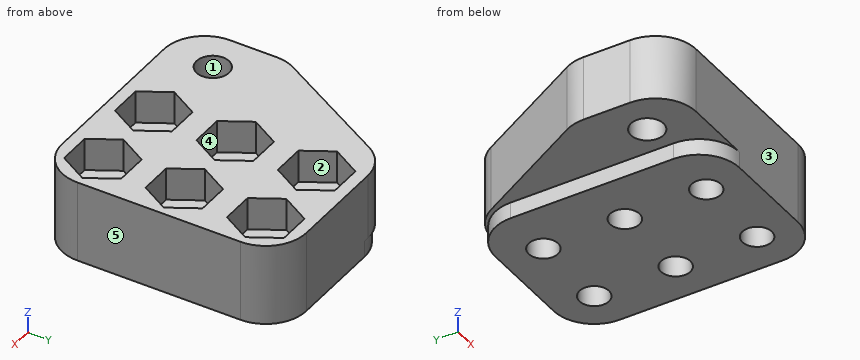
```python
from build123d import *

# Parameters (mm, degrees)
SKETCH1_R           = 2.286
SKETCH1_R_2         = 2.54
BOSS_EXTRUDE1_DEPTH = 12.7
FILLET1_R           = 6.35
CUT_EXTRUDE1_DEPTH  = 5.08
CUT_EXTRUDE2_START  = -2.54
SKETCH3_R           = 2.54
CUT_EXTRUDE2_DEPTH  = 2.54
FILLET2_R           = 6.35


with BuildPart() as part:
    # Sketch1 → Boss-Extrude1 (new body)
    with BuildSketch(Plane.XY):
        Polygon((-6.35, 31.75), (-19.05, 8.89), (-19.05, -6.35), (-6.35, -6.35), (19.05, -6.35), (19.05, 31.75), align=None)
        Circle(SKETCH1_R, mode=Mode.SUBTRACT)
        with Locations((-12.7, 1.27)):
            Circle(SKETCH1_R_2, mode=Mode.SUBTRACT)
        with Locations((12.7, 0)):
            Circle(SKETCH1_R, mode=Mode.SUBTRACT)
        with Locations((12.7, 12.7)):
            Circle(SKETCH1_R, mode=Mode.SUBTRACT)
        with Locations((12.7, 25.4)):
            Circle(SKETCH1_R, mode=Mode.SUBTRACT)
        with Locations((0, 12.7)):
            Circle(SKETCH1_R, mode=Mode.SUBTRACT)
        with Locations((0, 25.4)):
            Circle(SKETCH1_R, mode=Mode.SUBTRACT)
    extrude(amount=BOSS_EXTRUDE1_DEPTH)

    # Fillet1
    fillet1_edges = [part.edges().sort_by_distance(p)[0] for p in [
        (-19.05, -6.35, 6.35),
        (-19.05, 8.89, 6.35),
        (-6.35, 31.75, 6.35),
        (19.05, 31.75, 6.35),
        (19.05, -6.35, 6.35),
    ]]
    fillet(fillet1_edges, radius=FILLET1_R)

    # Sketch2 → Cut-Extrude1 (cut)
    with BuildSketch(Plane.XY.offset(12.7)):
        Polygon((17.832643893, 0), (15.266321947, 4.445), (10.133678053, 4.445), (7.567356107, 0), (10.133678053, -4.445), (15.266321947, -4.445), align=None)
        Polygon((5.132643893, 0), (2.566321947, 4.445), (-2.566321947, 4.445), (-5.132643893, 0), (-2.566321947, -4.445), (2.566321947, -4.445), align=None)
        Polygon((17.832643893, 12.7), (15.266321947, 17.145), (10.133678053, 17.145), (7.567356107, 12.7), (10.133678053, 8.255), (15.266321947, 8.255), align=None)
        Polygon((17.832643893, 25.4), (15.266321947, 29.845), (10.133678053, 29.845), (7.567356107, 25.4), (10.133678053, 20.955), (15.266321947, 20.955), align=None)
        Polygon((5.132643893, 12.7), (2.566321947, 17.145), (-2.566321947, 17.145), (-5.132643893, 12.7), (-2.566321947, 8.255), (2.566321947, 8.255), align=None)
        Polygon((5.132643893, 25.4), (2.566321947, 29.845), (-2.566321947, 29.845), (-5.132643893, 25.4), (-2.566321947, 20.955), (2.566321947, 20.955), align=None)
    extrude(amount=-CUT_EXTRUDE1_DEPTH, mode=Mode.SUBTRACT)

    # Sketch3 → Cut-Extrude2 (cut)
    with BuildSketch(Plane(origin=(0, 0, 0), x_dir=(-1, 0, 0), z_dir=(0, 0, -1)).offset(CUT_EXTRUDE2_START)):
        with BuildLine():
            Line((18.250898703, 10.328382334), (8.164537437, 28.483832613))
            Line((8.164537437, 28.483832613), (8.164537437, -6.35))
            Line((8.164537437, -6.35), (12.7, -6.35))
            ThreePointArc((12.7, -6.35), (17.190128061, -4.490128061), (19.05, 0))
            Line((19.05, 0), (19.05, 7.244549721))
            ThreePointArc((19.05, 7.244549721), (18.846979208, 8.837392029), (18.250898703, 10.328382334))
        make_face()
        with Locations((12.7, 1.27)):
            Circle(SKETCH3_R, mode=Mode.SUBTRACT)
    extrude(amount=CUT_EXTRUDE2_DEPTH, mode=Mode.SUBTRACT)

    # Fillet2
    # the kernel refuses this fillet: 6.35 mm, written as the material it takes off along each edge
    with BuildSketch(Plane(origin=(-8.164537437, -6.35, 2.54), x_dir=(1, 0, 0), z_dir=(0, 0, -1))) as fillet2_piece_1:
        with BuildLine():
            CenterArc((FILLET2_R, -FILLET2_R), FILLET2_R, 90, 90)
            Line((0, -FILLET2_R), (0, 0))
            Line((0, 0), (FILLET2_R, 0))
        make_face()
    extrude(amount=18.415, mode=Mode.SUBTRACT)
    with BuildSketch(Plane(origin=(-8.164537437, 28.483832613, -17.851881799), x_dir=(0.8892619937285123, 0.45739819250844366, 0), z_dir=(0, 0, 1))) as fillet2_piece_2:
        with BuildLine():
            CenterArc((4.236274197, -5.64681366), FILLET2_R, 62.780655364, 90)
            Line((-1.410539463, -2.742335138), (-1.975220829, -2.451887286))
            Line((-1.975220829, -2.451887286), (-0.564681366, 0.290447852))
            Line((-0.564681366, 0.290447852), (-0.352566378, 0.528130617))
            ThreePointArc((-0.352566378, 0.528130617), (6.720590159, 0.930188855), (7.431200572, 0.564681366))
            Line((7.431200572, 0.564681366), (7.140752719, 0))
        make_face()
    extrude(amount=20.391881799, mode=Mode.SUBTRACT)


solid = part.part
```
Verification items for the finished model (mm, model axes). Face numbers are marked on the shaded views. A direction names the side the tool comes from. Coordinates: 2 decimals unless noted, no trailing zeros. Order: outer loops, then holes, each group sorted by start corner. A loop starts at its lowest first (then second) coordinate and runs counter-clockwise, first axis right, second up. Notation, with made-up numbers: (14, 59.5) - (36, 59.5) arc R20 cw to (36, 86.5) - close; hole circle Ø2 at (64, 38.25). An arc over 180 degrees is marked (long way). Return JSON: item names as keys, results as strings.
(1) Go/stop test with flat-tipped pins: pin 1 (1 mm diameter, centred on y = 13.5, z = 7.5, fed in from -X); pin 2 (6 mm diameter, centred on x = 0, y = 12.7, fed in from +Z); pin 3 (0.8 mm diameter, centred on y = 9.5, z = 1.5, fed in from -X). Record where each tip stops, or that it passes through.
Filled sheet:
{"pin 1": "stops at x = -16.77", "pin 2": "stops at z = 7.62", "pin 3": "stops at x = -8.16"}
(2) Access from +Z, -Z, +X, -X, +Y, -Y to the whole of each face (thin tool, end or side, straight path). Record for the marked faces 1 and 2.
Filled sheet:
{"face 1": "+Z, -Z", "face 2": "+Z"}
(3) Section check B-B, the plane y = 13.5. Record the cut outline in (x, z), and give its area (3 significant figures).
Filled sheet:
{"outline": "(-16.49, 2.54) - (-8.16, 2.54) - (-8.16, 0) - (-2.14, 0) - (-2.14, 7.62) - (-4.67, 7.62) - (-4.67, 12.7) - (-16.49, 12.7) - close; (2.14, 0) - (10.56, 0) - (10.56, 7.62) - (8.03, 7.62) - (8.03, 12.7) - (4.67, 12.7) - (4.67, 7.62) - (2.14, 7.62) - close; (14.84, 0) - (19.05, 0) - (19.05, 12.7) - (17.37, 12.7) - (17.37, 7.62) - (14.84, 7.62) - close", "area": "270 mm^2"}
(4) Mould release check, pull along Y, two halves, no side actions. Record for the marked faces 3, 4 and 5: pulls with the +Y half, pulls with the -Y half, needs draft (parallel to the pull), parting line crosses it, or undercut.
Filled sheet:
{"face 3": "pulls with the -Y half", "face 4": "undercut", "face 5": "needs draft"}
(5) Thickness scan on line 1 along Y through (x, z) = (0, 2); line 2 along X through (y, z) = (12.7, 4); line 3 along X through (y, z) = (26.5, 0.75). Record the ranges inside material, lowest first.
Filled sheet:
{"line 1": "y = -6.35 to -2.29, 2.29 to 10.41, 14.99 to 23.11, 27.69 to 31.75", "line 2": "x = -16.93 to -2.29, 2.29 to 10.41, 14.99 to 19.05", "line 3": "x = -8.07 to -2, 2 to 10.7, 14.7 to 18.95"}
(6) Section check C-C, the plane z = 1.75. Record the cut outline in (x, y).
Filled sheet:
{"outline": "(-8.16, 0) arc R6.35 ccw to (-1.81, -6.35) - (12.7, -6.35) arc R6.35 ccw to (19.05, 0) - (19.05, 25.4) arc R6.35 ccw to (12.7, 31.75) - (-1.81, 31.75) arc R6.35 ccw to (-8.16, 25.4) - close; hole circle Ø4.57 at (0, 0); hole circle Ø4.57 at (0, 12.7); hole circle Ø4.57 at (0, 25.4); hole circle Ø4.57 at (12.7, 0); hole circle Ø4.57 at (12.7, 12.7); hole circle Ø4.57 at (12.7, 25.4)"}
(7) Section check A-A, the plane z = 5.75. Record the cut outline in (x, y).
Filled sheet:
{"outline": "(-19.05, 0) arc R6.35 ccw to (-12.7, -6.35) - (12.7, -6.35) arc R6.35 ccw to (19.05, 0) - (19.05, 25.4) arc R6.35 ccw to (12.7, 31.75) - (-2.61, 31.75) arc R6.35 ccw to (-8.16, 28.48) - (-18.25, 10.33) arc R6.35 ccw to (-19.05, 7.24) - close; hole circle Ø5.08 at (-12.7, 1.27); hole circle Ø4.57 at (0, 0); hole circle Ø4.57 at (0, 12.7); hole circle Ø4.57 at (0, 25.4); hole circle Ø4.57 at (12.7, 0); hole circle Ø4.57 at (12.7, 12.7); hole circle Ø4.57 at (12.7, 25.4)"}
(8) Section check D-D, the plane x = 11. Record the cut outline in (y, z) (3 decimals).
Filled sheet:
{"outline": "(-6.35, 0) - (-1.528, 0) - (-1.528, 7.62) - (-4.445, 7.62) - (-4.445, 12.7) - (-6.35, 12.7) - close; (1.528, 0) - (11.172, 0) - (11.172, 7.62) - (8.255, 7.62) - (8.255, 12.7) - (4.445, 12.7) - (4.445, 7.62) - (1.528, 7.62) - close; (14.228, 0) - (23.872, 0) - (23.872, 7.62) - (20.955, 7.62) - (20.955, 12.7) - (17.145, 12.7) - (17.145, 7.62) - (14.228, 7.62) - close; (26.928, 0) - (31.75, 0) - (31.75, 12.7) - (29.845, 12.7) - (29.845, 7.62) - (26.928, 7.62) - close"}
